Work out the finished part from the listing and answer in its coordinate system (mm). A direction names the side the tool comes from. Round coordinates to 2 decimals unless told otherwise and drop trailing zeros. Loops run counter-clockwise (first coordinate to the right, second up) from the corner with the lowest first, then second, coordinate; pieces in that order, holes last. Notation, with made-up numbers: (-19, 79.5) - (5, 79.5) arc R10 cw to (5, 83.5) - close; hole circle Ø2 at (63, 16.25). An arc over 180 degrees is marked (long way). Return JSON: item names as keys, results as strings.
from build123d import *

# Parameters (mm, degrees)
ESQUISSE1_W        = 28
ESQUISSE1_H        = 50
ESQUISSE1_W_2      = 20
ESQUISSE1_H_2      = 42
BOSS_EXTRU_1_DEPTH = 5
CONG_1_R           = 7


with BuildPart() as part:
    # Esquisse1 → Boss.-Extru.1 (new body)
    with BuildSketch(Plane(origin=(0, 0, 0), x_dir=(1, 0, 0), z_dir=(0, 1, 0))):
        Rectangle(ESQUISSE1_W, ESQUISSE1_H)
        Rectangle(ESQUISSE1_W_2, ESQUISSE1_H_2, mode=Mode.SUBTRACT)
    extrude(amount=BOSS_EXTRU_1_DEPTH)

    # Congé1
    cong_1_edges = [part.edges().sort_by_distance(p)[0] for p in [
        (14, 2.5, 25),
        (-14, 2.5, 25),
        (-14, 2.5, -25),
        (14, 2.5, -25),
    ]]
    fillet(cong_1_edges, radius=CONG_1_R)


solid = part.part
1) Find the intervals of material crossed by L1, parallel to X at y = 3.9, z = 16.5; L2, parallel to Z at x = -2.75, y = 2.7; L3, parallel to X at y = 3.5, z = 20.5, in increasing order.
Verdict:
{"L1": "x = -14 to -10, 10 to 14", "L2": "z = -25 to -21, 21 to 25", "L3": "x = -13.54 to -10, 10 to 13.54"}
2) Section A-A (z = -3) is taken. Give the vertices of the cut face in (x, y), and give its area (3 significant figures).
Verdict:
{"outline": "(-14, 0) - (-10, 0) - (-10, 5) - (-14, 5) - close; (10, 0) - (14, 0) - (14, 5) - (10, 5) - close", "area": "40.0 mm2"}
3) A tool of negligible diameter and unlimited length cuts with its end or side. For faces 1 (the cylindrical face through (-12, 2.5, -22.9)), 2 (the flat face through (-10, 2, 0)), from which of +Z, -Z, +X, -X, +Y, -Y can it reach the whole face along a straight path? Write none if from no direction.
Verdict:
{"face 1": "-Z, -X, +Y, -Y", "face 2": "+Y, -Y"}
4) Section D-D (x = 12) is taken. Give the vertices of the cut face in (y, z), and give its area (3 significant figures).
Verdict:
{"outline": "(0, -22.9) - (5, -22.9) - (5, 22.9) - (0, 22.9) - close", "area": "229 mm2"}
5) Section B-B (x = 1.75) is taken. Give the vertices of the cut face in (y, z).
Verdict:
{"outline": "(0, -25) - (5, -25) - (5, -21) - (0, -21) - close; (0, 21) - (5, 21) - (5, 25) - (0, 25) - close"}
6) Flat-ended cylindrical pins translate along their axes: pin 1 (3 mm diameter, centred on x = -9, y = 2, fed in from -Z); pin 2 (1.5 mm diameter, centred on x = 10.5, y = 2.5, fed in from -Z). Find the tip coordinate at first contact, or state that the pin passes through.
Verdict:
{"pin 1": "stops at z = -24.98", "pin 2": "stops at z = -24.44"}
7) Section C-C (y = 0.6) is taken. Give the vertices of the cut face in (x, z).
Verdict:
{"outline": "(-14, -18) arc R7 ccw to (-7, -25) - (7, -25) arc R7 ccw to (14, -18) - (14, 18) arc R7 ccw to (7, 25) - (-7, 25) arc R7 ccw to (-14, 18) - close; hole (-10, -21) - (10, -21) - (10, 21) - (-10, 21) - close"}
8) Determine the mould class of faces 3 (the cylindrical face through (11.9, 2.5, 23)), 4 (the cylindrical face through (-12, 2.5, 22.9)), 5 (the flat face through (0, 2, -21)) for opening direction X: pulls with the +X half, pulls with the -X half, needs draft (parallel to the pull), parting line crosses it, or undercut.
Verdict:
{"face 3": "pulls with the +X half", "face 4": "pulls with the -X half", "face 5": "undercut"}
